The model under review builds one solid part; all positions refer to its coordinate system, in mm. A direction names the side the tool comes from. Round coordinates to 2 decimals unless told otherwise and drop trailing zeros. Loops run counter-clockwise (first coordinate to the right, second up) from the corner with the lowest first, then second, coordinate; pieces in that order, holes last. Notation, with made-up numbers: M 3.5,79 L 20.5,79 A20 ccw 20.5,111 Z; hole C 70,-18 d3. An arc over 180 degrees is marked long. One line per question, with ' | ' between items.
from build123d import *

# Parameters (mm, degrees)
SKETCH1_R           = 6
BOSS_EXTRUDE1_DEPTH = 36
BOSS_EXTRUDE2_DEPTH = 8
SKETCH3_OUTSIDE_W   = 53.532
SKETCH3_OUTSIDE_H   = 51.488
SKETCH3_OUTSIDE_R   = 9.5
CUT_EXTRUDE1_DEPTH  = 8
CUT_EXTRUDE1_DRAFT  = -50
SKETCH4_OUTSIDE_W   = 53.532
SKETCH4_OUTSIDE_H   = 51.488
SKETCH4_OUTSIDE_R   = 9.5
CUT_EXTRUDE3_DEPTH  = 8
CUT_EXTRUDE3_DRAFT  = -50
BOSS_EXTRUDE3_DEPTH = 8
SKETCH6_OUTSIDE_W   = 54.894
SKETCH6_OUTSIDE_H   = 52.85
SKETCH6_OUTSIDE_R   = 9.5
CUT_EXTRUDE6_DEPTH  = 8
CUT_EXTRUDE6_DRAFT  = -50
SKETCH7_OUTSIDE_W   = 54.894
SKETCH7_OUTSIDE_H   = 52.85
SKETCH7_OUTSIDE_R   = 9.481063721
CUT_EXTRUDE7_DEPTH  = 8
CUT_EXTRUDE7_DRAFT  = -50


with BuildPart() as part:
    # Sketch1 → Boss-Extrude1 (new body)
    with BuildSketch(Plane.XY):
        Circle(SKETCH1_R)
    extrude(amount=BOSS_EXTRUDE1_DEPTH)

    # Sketch2 → Boss-Extrude2 (add)
    with BuildSketch(Plane(origin=(0, 0, 0), x_dir=(-1, 0, 0), z_dir=(0, 0, -1))):
        Polygon((-10.93381737, 0.885985919), (-6.234194998, -9.025970644), (4.699622372, -9.911956562), (10.93381737, -0.885985919), (6.234194998, 9.025970644), (-4.699622372, 9.911956562), align=None)
    extrude(amount=BOSS_EXTRUDE2_DEPTH)


with BuildPart() as cut_extrude1_tool:
    # Sketch3 outside → Cut-Extrude1 (with draft: the straight prism first)
    with BuildSketch(Plane.XY):
        Rectangle(SKETCH3_OUTSIDE_W, SKETCH3_OUTSIDE_H)
        Circle(SKETCH3_OUTSIDE_R, mode=Mode.SUBTRACT)
    extrude(amount=-CUT_EXTRUDE1_DEPTH)
    # Cut-Extrude1: the draft: its side faces are tilted about the plane it starts from
    cut_extrude1_sides = [cut_extrude1_tool.faces().sort_by_distance(p)[0] for p in [
        (0, -25.744, -4),
        (26.766, 0, -4),
        (0, 25.744, -4),
        (-26.766, 0, -4),
        (-9.5, 0, -4),
    ]]
    draft(cut_extrude1_sides, Plane.XY, CUT_EXTRUDE1_DRAFT)


with BuildPart() as part_1:
    add(part.part)

    # Cut-Extrude1: cut by cut_extrude1_tool
    add(cut_extrude1_tool.part, mode=Mode.SUBTRACT)


with BuildPart() as cut_extrude3_tool:
    # Sketch4 outside → Cut-Extrude3 (with draft: the straight prism first)
    with BuildSketch(Plane(origin=(0, 0, -8), x_dir=(-1, 0, 0), z_dir=(0, 0, -1))):
        Rectangle(SKETCH4_OUTSIDE_W, SKETCH4_OUTSIDE_H)
        Circle(SKETCH4_OUTSIDE_R, mode=Mode.SUBTRACT)
    extrude(amount=-CUT_EXTRUDE3_DEPTH)
    # Cut-Extrude3: the draft: its side faces are tilted about the plane it starts from
    cut_extrude3_sides = [cut_extrude3_tool.faces().sort_by_distance(p)[0] for p in [
        (0, -25.744, -4),
        (-26.766, 0, -4),
        (0, 25.744, -4),
        (26.766, 0, -4),
        (9.5, 0, -4),
    ]]
    draft(cut_extrude3_sides, Plane(origin=(0, 0, -8), x_dir=(-1, 0, 0), z_dir=(0, 0, -1)), CUT_EXTRUDE3_DRAFT)


with BuildPart() as part_2:
    add(part_1.part)

    # Cut-Extrude3: cut by cut_extrude3_tool
    add(cut_extrude3_tool.part, mode=Mode.SUBTRACT)

    # Sketch5 → Boss-Extrude3 (add)
    with BuildSketch(Plane.XY.offset(36)):
        Polygon((-6.252986911, 8.986336688), (-10.908889314, -0.92207717), (-4.655902404, -9.908413858), (6.252986911, -8.986336688), (10.908889314, 0.92207717), (4.655902404, 9.908413858), align=None)
    extrude(amount=BOSS_EXTRUDE3_DEPTH)


with BuildPart() as cut_extrude6_tool:
    # Sketch6 outside → Cut-Extrude6 (with draft: the straight prism first)
    with BuildSketch(Plane(origin=(0, 0, 36), x_dir=(-1, 0, 0), z_dir=(0, 0, -1))):
        Rectangle(SKETCH6_OUTSIDE_W, SKETCH6_OUTSIDE_H)
        Circle(SKETCH6_OUTSIDE_R, mode=Mode.SUBTRACT)
    extrude(amount=-CUT_EXTRUDE6_DEPTH)
    # Cut-Extrude6: the draft: its side faces are tilted about the plane it starts from
    cut_extrude6_sides = [cut_extrude6_tool.faces().sort_by_distance(p)[0] for p in [
        (0, -26.425, 40),
        (-27.447, 0, 40),
        (0, 26.425, 40),
        (27.447, 0, 40),
        (9.5, 0, 40),
    ]]
    draft(cut_extrude6_sides, Plane(origin=(0, 0, 36), x_dir=(-1, 0, 0), z_dir=(0, 0, -1)), CUT_EXTRUDE6_DRAFT)


with BuildPart() as part_3:
    add(part_2.part)

    # Cut-Extrude6: cut by cut_extrude6_tool
    add(cut_extrude6_tool.part, mode=Mode.SUBTRACT)


with BuildPart() as cut_extrude7_tool:
    # Sketch7 outside → Cut-Extrude7 (with draft: the straight prism first)
    with BuildSketch(Plane.XY.offset(44)):
        Rectangle(SKETCH7_OUTSIDE_W, SKETCH7_OUTSIDE_H)
        Circle(SKETCH7_OUTSIDE_R, mode=Mode.SUBTRACT)
    extrude(amount=-CUT_EXTRUDE7_DEPTH)
    # Cut-Extrude7: the draft: its side faces are tilted about the plane it starts from
    cut_extrude7_sides = [cut_extrude7_tool.faces().sort_by_distance(p)[0] for p in [
        (0, -26.425, 40),
        (27.447, 0, 40),
        (0, 26.425, 40),
        (-27.447, 0, 40),
        (-9.481063721, 0, 40),
    ]]
    draft(cut_extrude7_sides, Plane.XY.offset(44), CUT_EXTRUDE7_DRAFT)


with BuildPart() as part_4:
    add(part_3.part)

    # Cut-Extrude7: cut by cut_extrude7_tool
    add(cut_extrude7_tool.part, mode=Mode.SUBTRACT)


solid = part_4.part
1) For line 1 (Z direction, x = 3, y = 7); line 2 (Y direction, x = 0, z = 15); line 3 (X direction, y = 5.25, z = 24), list the stretches that pass through material, from the lowest coordinate up.
Output values:
line 1: z = -8 to 0, 36 to 44 | line 2: y = -6 to 6 | line 3: x = -2.9 to 2.9
2) Insertion check: P1, Ø4, axis at y = 6.5, z = 24.5, coming from the -X side; P2, Ø2, axis at x = 4.5, z = 25, coming from the -Y side; P3, Ø3, axis at y = -5.5, z = 5, coming from the +X side. Each pin has a flat end and moves straight along its axis. Give the tip position at first contact, or say it passes through.
Output values:
P1: stops at x = -3.97 | P2: stops at y = -4.87 | P3: stops at x = 4.47
3) Machinability: for faces 4 (the flat face through (-0.1, -6.2, 36)), 5 (the conical face through (9.82, 0.772, -0.294)), 6 (the conical face through (5.61, -8.025, 36.245)), 7 (the flat face through (-8.55, 4.1, 39.94)), which of the approach directions +Z, -Z, +X, -X, +Y, -Y give a long, thin tool a straight path to every point of the face, cutting with its end or side? Answer none if there is none.
Output values:
face 4: none | face 5: +X | face 6: +X, -Y | face 7: +Z, -X, +Y
4) Add section B-B on z = 14. State the section outline as (x, y) points, then the cut area to 3 significant figures.
Output values:
outline: C 0,0 d12 | area: 113 mm²
5) Mouldability with a two-part tool opening along Z and no side actions: class faces 1 (the flat face through (0, 0, 44)), 2 (the conical face through (5.618, -8.091, -7.706)), 3 (the conical face through (-4.145, -8.871, 36.245)) as +Z half, -Z half, draft (parallel to the pull), parting line (faces both ways), or undercut.
Output values:
face 1: +Z half | face 2: -Z half | face 3: undercut
6) Add section A-A on y = 0. State the section outline as (x, z) points, then the cut area to 3 significant figures.
Output values:
outline: M -10.51,-7.15 L -9.5,-8 L 9.5,-8 L 10.51,-7.15 L 10.51,-0.85 L 9.5,0 L 6,0 L 6,36 L 9.5,36 L 10.48,36.82 L 10.48,43.17 L 9.48,44 L -9.48,44 L -10.48,43.17 L -10.48,36.82 L -9.5,36 L -6,36 L -6,0 L -9.5,0 L -10.51,-0.85 Z | area: 764 mm²
